from build123d import *

# Parameters (mm, degrees)
SKETCH1_W      = 16
SKETCH1_H      = 71.4
BODY_DEPTH     = 5
SKETCH2_R      = 4
TOP_HOLE_DEPTH = 11


with BuildPart() as part:
    # Sketch1 → Body (new body, symmetric)
    with BuildSketch(Plane.XY):
        Rectangle(SKETCH1_W, SKETCH1_H)
    extrude(amount=BODY_DEPTH, both=True)

    # Sketch2 → Top Hole (cut, through all)
    with BuildSketch(Plane.XY.offset(5)):
        with Locations((0, 27.7)):
            Circle(SKETCH2_R)
    top_hole = extrude(amount=-TOP_HOLE_DEPTH, mode=Mode.SUBTRACT)

    # Bottom Hole: Top Hole across plane
    add(top_hole.mirror(Plane.ZX), mode=Mode.SUBTRACT)


solid = part.part
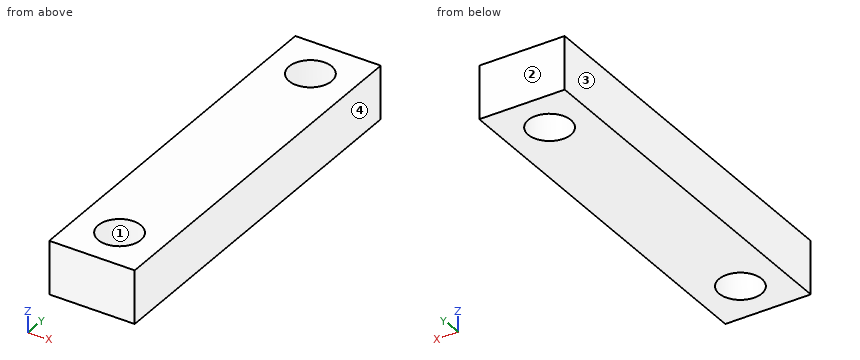
Geometry check sheet. Reference: the model listing, model coordinates, mm. Face numbers are marked on the shaded views. Round coordinates to 2 decimals unless told otherwise and drop trailing zeros. Order: outer loops, then holes, each group sorted by start corner. A loop starts at its lowest first (then second) coordinate and runs counter-clockwise, first axis right, second up. Notation, with made-up numbers: M -16,81 L -9,81 A15 cw -9,108 Z; hole C -9,13.5 d11. An arc over 180 degrees is marked long. Write each question's results on one line, items separated by ' | '. Start each with the question number.
1. Cross-section at B-B on y = 27.7. Record the boundary of the cut face in (x, z), plus the area to 3 significant figures.
2. Draft check along X on the marked faces 1, 2, 3 and 4. Enter one of: pulls with the +X half, pulls with the -X half, needs draft (parallel to the pull), parting line crosses it, or undercut.
3. Material ranges on L1, parallel to Y at x = 0, z = 2; L2, parallel to X at y = -27.7, z = -1.5; L3, parallel to Y at x = -2, z = 4, recorded low to high. Write a range as from..to.
4. Cross-section at A-A on x = 0. Record the boundary of the cut face in (y, z), plus the area to 3 significant figures.
5. Cross-section at C-C on z = 1. Record the boundary of the cut face in (x, y), plus the area to 3 significant figures.
Resolved:
1) outline: M -8,-5 L -4,-5 L -4,5 L -8,5 Z; M 4,-5 L 8,-5 L 8,5 L 4,5 Z | area: 80.0 mm2
2) face 1: undercut | face 2: needs draft | face 3: pulls with the -X half | face 4: pulls with the +X half
3) L1: -35.7..-31.7, -23.7..23.7, 31.7..35.7 | L2: -8..-4, 4..8 | L3: -35.7..-31.16, -24.24..24.24, 31.16..35.7
4) outline: M -35.7,-5 L -31.7,-5 L -31.7,5 L -35.7,5 Z; M -23.7,-5 L 23.7,-5 L 23.7,5 L -23.7,5 Z; M 31.7,-5 L 35.7,-5 L 35.7,5 L 31.7,5 Z | area: 554 mm2
5) outline: M -8,-35.7 L 8,-35.7 L 8,35.7 L -8,35.7 Z; hole C 0,-27.7 d8; hole C 0,27.7 d8 | area: 1,040 mm2
